Input: part model. Units: mm. Frame: model coordinates. A direction names the side the tool comes from. Give positions to 0.01 mm unless a question says otherwise; leave off trailing zeros. Order: outer loops, then holes, each group sorted by start corner. A loop starts at its lowest first (then second) coordinate and runs counter-clockwise, first axis right, second up. Notation, with made-up numbers: M 9.5,-26 L 50.5,-26 A31 ccw 50.5,4 Z; hole C -20,-29.5 d3. An arc over 180 degrees is marked long. Use a Markdown table: item, result.
from build123d import *

# Parameters (mm, degrees)
SKETCH1_W           = 511.53
SKETCH1_H           = 486.32
BOSS_EXTRUDE1_DEPTH = 150
SHELL1_T            = -10
SKETCH2_R           = 21
BOSS_EXTRUDE2_DEPTH = 90
SCALE1_SCALE        = 0.1
SCALE2_SCALE        = 3


with BuildPart() as part:
    # Sketch1 → Boss-Extrude1 (new body)
    with BuildSketch(Plane(origin=(0, 0, 0), x_dir=(1, 0, 0), z_dir=(0, 1, 0))):
        Rectangle(SKETCH1_W, SKETCH1_H)
    extrude(amount=BOSS_EXTRUDE1_DEPTH)

    # Shell1
    shell1_openings = [part.faces().sort_by_distance(p)[0] for p in [
        (0, 150, 0),
    ]]
    offset(amount=SHELL1_T, openings=shell1_openings, kind=Kind.INTERSECTION)

    # Sketch2 → Boss-Extrude2 (add)
    with BuildSketch(Plane(origin=(0, 10, 0), x_dir=(1, 0, 0), z_dir=(0, 1, 0))):
        with Locations(Location((0, 0, 0), (0, 0, 90))):
            Circle(SKETCH2_R)
    extrude(amount=BOSS_EXTRUDE2_DEPTH)


with BuildPart() as part_1:
    # Scale1: scaled about (0, 0, 0)
    add(part.part.scale(SCALE1_SCALE))


with BuildPart() as part_2:
    # Scale2: scaled about (0, 0, 0)
    add(part_1.part.scale(SCALE2_SCALE))


solid = part_2.part
1) Mould query, pull axis X, two halves, no side actions, for faces 1 (the face through (-73.73, 24, 1)), 2 (the face through (-76.73, 22, 1)), 3 (the face through (-34, 45, -71)). Classes: released by +X, released by -X, zero draft, split by the parting line, or undercut.
Response values:
| item | result |
|---|---|
| face 1 | undercut |
| face 2 | released by -X |
| face 3 | zero draft |
2) Cut plane A-A on y = 5. Return loops of the section in (x, z), and give its area (3 significant figures).
Response values:
| item | result |
|---|---|
| outline | M -76.73,-72.95 L 76.73,-72.95 L 76.73,72.95 L -76.73,72.95 Z; C 0,0 d12.6; hole M -73.73,-69.95 L 73.73,-69.95 L 73.73,69.95 L -73.73,69.95 Z |
| area | 1,880 mm² |
3) Cut plane C-C on z = 44. Return loops of the section in (x, y).
Response values:
| item | result |
|---|---|
| outline | M -76.73,0 L 76.73,0 L 76.73,45 L 73.73,45 L 73.73,3 L -73.73,3 L -73.73,45 L -76.73,45 Z |
4) Material intervals for line 1 (X direction, y = 25, z = -56); line 2 (X direction, y = 21.5, z = 2.5); line 3 (Z direction, x = 41.5, y = 30), sorted ascending. Write a range as from..to.
Response values:
| item | result |
|---|---|
| line 1 | x = -76.73..-73.73, 73.73..76.73 |
| line 2 | x = -76.73..-73.73, -5.78..5.78, 73.73..76.73 |
| line 3 | z = -72.95..-69.95, 69.95..72.95 |
5) Reachability of faces 4 (the face through (-1, 22, -72.948)), 5 (the face through (-1, 24, -69.948)) from +Z, -Z, +X, -X, +Y, -Y: full face, straight path, thin tool, end or side. Return the list, or none.
Response values:
| item | result |
|---|---|
| face 4 | -Z, +X, -X, +Y, -Y |
| face 5 | +Y |
6) Cut plane D-D on z = 0. Return loops of the section in (x, y), and give its area (3 significant figures).
Response values:
| item | result |
|---|---|
| outline | M -76.73,0 L 76.73,0 L 76.73,45 L 73.73,45 L 73.73,3 L 6.3,3 L 6.3,30 L -6.3,30 L -6.3,3 L -73.73,3 L -73.73,45 L -76.73,45 Z |
| area | 1,050 mm² |
7) Cut plane B-B on x = -13.5. Return loops of the section in (y, z).
Response values:
| item | result |
|---|---|
| outline | M 0,-72.95 L 45,-72.95 L 45,-69.95 L 3,-69.95 L 3,69.95 L 45,69.95 L 45,72.95 L 0,72.95 Z |
8) First-contact query: pin 1 Ø4 at (x, z) = (1.5, -0.5) entering from +Y. Flat tip, straight axial feed; report the tip coordinate or a pass-through.
Response values:
| item | result |
|---|---|
| pin 1 | stops at y = 30 |
